Design review of the part built by this model. Coordinates are the model's own, in mm. A direction names the side the tool comes from. Give positions to 0.01 mm unless a question says otherwise; leave off trailing zeros. Write each loop counter-clockwise with the first axis right and the second up, starting at its lowest first coordinate (ties: lowest second). Pieces come first, ordered by that corner, then holes. Notation, with made-up numbers: M -3,-1.75 L 17,-1.75 A26 ccw 17,26.25 Z; hole C 66.5,66 d11. An arc over 180 degrees is marked long. Use one line per item in the form item = value. Start each with the question number.
from build123d import *

# Parameters (mm, degrees)
SKETCH2_R           = 1.5
BOSS_EXTRUDE1_DEPTH = 6.4


with BuildPart() as part:
    # Sketch2 → Boss-Extrude1 (new body)
    with BuildSketch(Plane.XY):
        Polygon((35.75, 58.5), (110.75, 58.5), (110.75, 74.92), (143.58, 74.92), (146.5, 72), (146.5, 65.999038761), (136, 65.999038761), (136, 67.249038761), (134.2, 67.249038761), (134.2, 65.999038761), (132.8, 65.999038761), (132.8, 62.999320414), (134.2, 62.999320414), (134.2, 61.749320414), (136, 61.749320414), (136, 62.999320414), (146.5, 62.999320414), (146.5, 60.13073157), (140.5, 59.88073157), (140.5, 57.18073157), (146.5, 56.88073157), (146.5, 50.13073157), (140.5, 49.83073157), (140.5, 47.13073157), (146.5, 46.88073157), (146.5, 35.499320414), (136, 35.499320414), (136, 36.749320414), (134.2, 36.749320414), (134.2, 35.499320414), (132.8, 35.499320414), (132.8, 32.499602067), (134.2, 32.499602067), (134.2, 31.249602067), (136, 31.249602067), (136, 32.499602067), (146.5, 32.499602067), (146.5, 21.11926843), (140.5, 20.86926843), (140.5, 18.16926843), (146.5, 17.86926843), (146.5, 11.11926843), (140.5, 10.81926843), (140.5, 8.11926843), (146.5, 7.86926843), (146.5, 0), (138, 0), (138, 1.5), (133.2, 1.5), (133.2, 0), (128.3, 0), (128.025, -5.5), (118.325, -5.5), (118.05, 0), (114.75, 0), (114.75, 7.7), (116, 7.7), (116, 9.5), (114.75, 9.5), (114.75, 10.9), (111.750281653, 10.9), (111.750281653, 9.5), (110.500281653, 9.5), (110.500281653, 7.7), (111.750281653, 7.7), (111.750281653, 0), (97.3, 0), (97.025, -5.5), (87.325, -5.5), (87.05, 0), (79.85, 0), (79.85, 4.5), (66.65, 4.5), (66.65, 0), (59.45, 0), (59.175, -5.5), (49.475, -5.5), (49.2, 0), (34.749718347, 0), (34.749718347, 7.7), (35.999718347, 7.7), (35.999718347, 9.5), (34.749718347, 9.5), (34.749718347, 10.9), (31.75, 10.9), (31.75, 9.5), (30.5, 9.5), (30.5, 7.7), (31.75, 7.7), (31.75, 0), (28.45, 0), (28.175, -5.5), (18.475, -5.5), (18.2, 0), (13.3, 0), (13.3, 1.5), (8.5, 1.5), (8.5, 0), (0, 0), (0, 7.86926843), (6, 8.11926843), (6, 10.81926843), (0, 11.11926843), (0, 17.86926843), (6, 18.16926843), (6, 20.86926843), (0, 21.11926843), (0, 32.499602067), (10.5, 32.499602067), (10.5, 31.249602067), (12.3, 31.249602067), (12.3, 32.499602067), (13.7, 32.499602067), (13.7, 35.499320414), (12.3, 35.499320414), (12.3, 36.749320414), (10.5, 36.749320414), (10.5, 35.499320414), (0, 35.499320414), (0, 46.88073157), (6, 47.13073157), (6, 49.83073157), (0, 50.13073157), (0, 56.88073157), (6, 57.18073157), (6, 59.88073157), (0, 60.13073157), (0, 62.999320414), (10.5, 62.999320414), (10.5, 61.749320414), (12.3, 61.749320414), (12.3, 62.999320414), (13.7, 62.999320414), (13.7, 65.999038761), (12.3, 65.999038761), (12.3, 67.249038761), (10.5, 67.249038761), (10.5, 65.999038761), (0, 65.999038761), (0, 72), (2.92, 74.92), (35.75, 74.92), align=None)
        with Locations((31.25, 46.866359173)):
            Circle(SKETCH2_R, mode=Mode.SUBTRACT)
        with Locations(Location((115.25, 46.866359173, 0), (0, 0, 180))):
            Circle(SKETCH2_R, mode=Mode.SUBTRACT)
    extrude(amount=BOSS_EXTRUDE1_DEPTH)


solid = part.part
1. Clearance check with flat-ended pins moving along their axes: pin 1 Ø2 at (x, y) = (20.5, 33.5) entering from -Z; pin 2 Ø1.4 at (x, z) = (11.5, 2) entering from -Y; pin 3 Ø0.8 at (y, z) = (58, 4.5) entering from +X. State where each tip first meets the part, or that it passes through.
2. Draft analysis for pull direction X (two halves, no side actions). For faces 6 (the flat face through (128.164, -2.712, 3.155)), 7 (the flat face through (3.042, 20.993, 3.155)), 8 (the flat face through (31.75, 4, 3)), 9 (the flat face through (59.314, -2.712, 3.155)), state which applies: pulls with the +X half, pulls with the -X half, needs draft (parallel to the pull), parting line crosses it, or undercut.
3. To check wall thickness, follow L1, parallel to Y at x = 115.25, z = 4.25; L2, parallel to X at y = 62, z = 6; L3, parallel to X at y = 71.5, z = 4.5. State the ranges of each line that lie inside material, in increasing order.
4. We need section A-A (x = 68). State the section outline as (y, z) points, and give its area (3 significant figures).
5. We need section B-B (z = 2.5). Give the number of separate pieces and of enclosed holes in the cut face, and give its area (3 significant figures).
6. For faces 1 (the flat face through (116, 0, 3)), 2 (the flat face through (141, 35.499, 3)), 3 (the flat face through (2.958, 18.017, 3.155)), 4 (the flat face through (1, 73, 3)), 5 (the flat face through (4, 0, 3)), list the 3-axis set-ups (+Z, -Z, +X, -X, +Y, -Y) from which the entire face can be reached by the end or side of a thin tool; tool diameter is ignored.
7. We need section C-C (y = 34). State the section outline as (x, z) points, and give its area (3 significant figures).
Answer block:
q1.pin_1 = 0
q1.pin_2 = 1.5
q1.pin_3 = 140.5
q2.face_6 = pulls with the +X half
q2.face_7 = pulls with the -X half
q2.face_8 = undercut
q2.face_9 = undercut
q3.L1 = 0 to 7.7, 9.5 to 45.37, 48.37 to 74.92
q3.L2 = 0 to 10.5, 12.3 to 35.75, 110.75 to 134.2, 136 to 146.5
q3.L3 = 0 to 35.75, 110.75 to 146.5
q4.outline = M 4.5,0 L 58.5,0 L 58.5,6.4 L 4.5,6.4 Z
q4.area = 346 mm^2
q5.separate_pieces = 1
q5.enclosed_holes = 2
q5.area = 9,470 mm^2
q6.face_1 = +Z, -Z, -Y
q6.face_2 = +Z, -Z, +X
q6.face_3 = +Z, -Z, -X
q6.face_4 = +Z, -Z, -X, +Y
q6.face_5 = +Z, -Z, -X, -Y
q7.outline = M 13.7,0 L 132.8,0 L 132.8,6.4 L 13.7,6.4 Z
q7.area = 762 mm^2
